```python
from build123d import *

# Parameters (mm, degrees)
F1_DEPTH = 5
F2_R     = 12.5
F3_DEPTH = 3
F3_TAPER = 30
F4_R     = 7.5
F5_DEPTH = 5.0010001
F6_DEPTH = 5.0010001
F7_R     = 3


# Not quite as in the source:
# - a pattern or mirror of a feature is missing from the dataset's text; its kind, count and spacing are read off the source's solid


with BuildPart() as f1:
    # F0 (on Front) → F1 (new body, symmetric)
    with BuildSketch(Plane.XZ):
        with BuildLine():
            ThreePointArc((19.8138622769, -2.7222897845), (19.9534113066, -1.3643229935), (20, 0))
            ThreePointArc((20, 0), (16.5979995869, 11.1582440246), (7.5493590287, 18.5204529711))
            Line((7.5493590287, 18.5204529711), (-7.5493590287, 18.5204529711))
            ThreePointArc((-7.5493590287, 18.5204529711), (-17.3205080757, 10), (-19.8138622769, -2.7222897845))
            Line((-19.8138622769, -2.7222897845), (-12.2645032483, -15.7981631867))
            ThreePointArc((-12.2645032483, -15.7981631867), (0, -20), (12.2645032483, -15.7981631867))
            Line((12.2645032483, -15.7981631867), (19.8138622769, -2.7222897845))
        make_face()
        with BuildLine():
            Line((-7.5493590287, 18.5204529711), (7.5493590287, 18.5204529711))
            ThreePointArc((7.5493590287, 18.5204529711), (0, 20), (-7.5493590287, 18.5204529711))
        make_face()
        with BuildLine():
            ThreePointArc((-7.5493590287, 18.5204529711), (0, 20), (7.5493590287, 18.5204529711))
            Line((7.5493590287, 18.5204529711), (7.5493590287, 42.3402367583))
            Line((7.5493590287, 42.3402367583), (-7.5493590287, 42.3402367583))
            Line((-7.5493590287, 42.3402367583), (-7.5493590287, 18.5204529711))
        make_face()
        with BuildLine():
            Line((40.4424001493, -14.632181678), (19.8138622769, -2.7222897845))
            ThreePointArc((19.8138622769, -2.7222897845), (17.3205080757, -10), (12.2645032483, -15.7981631867))
            Line((12.2645032483, -15.7981631867), (32.8930411206, -27.7080550803))
            Line((32.8930411206, -27.7080550803), (40.4424001493, -14.632181678))
        make_face()
        with BuildLine():
            ThreePointArc((12.2645032483, -15.7981631867), (17.3205080757, -10), (19.8138622769, -2.7222897845))
            Line((19.8138622769, -2.7222897845), (12.2645032483, -15.7981631867))
        make_face()
        with BuildLine():
            Line((-12.2645032483, -15.7981631867), (-19.8138622769, -2.7222897845))
            ThreePointArc((-19.8138622769, -2.7222897845), (-17.3205080757, -10), (-12.2645032483, -15.7981631867))
        make_face()
        with BuildLine():
            ThreePointArc((-12.2645032483, -15.7981631867), (-17.3205080757, -10), (-19.8138622769, -2.7222897845))
            Line((-19.8138622769, -2.7222897845), (-40.4424001493, -14.632181678))
            Line((-40.4424001493, -14.632181678), (-32.8930411206, -27.7080550803))
            Line((-32.8930411206, -27.7080550803), (-12.2645032483, -15.7981631867))
        make_face()
    extrude(amount=F1_DEPTH, both=True)

    # F2 (on face) → F3 (cut)
    with BuildSketch(Plane(origin=(0, 5, 0), x_dir=(-1, 0, 0), z_dir=(0, 1, 0))):
        Circle(F2_R)
    f3 = extrude(amount=-F3_DEPTH, taper=F3_TAPER, mode=Mode.SUBTRACT)

    # F3_copies: F3 across plane
    add(f3.mirror(Plane(origin=(0, 0, 0), x_dir=(0, 0, -1), z_dir=(0, -1, 0))), mode=Mode.SUBTRACT)

    # F4 (on Front) → F5 (cut, through all)
    with BuildSketch(Plane.XZ):
        Circle(F4_R)
    extrude(amount=-F5_DEPTH, mode=Mode.SUBTRACT)

    # F6 (cut, through all): a face of the model
    f6_faces = [f1.faces().sort_by_distance(p)[0] for p in [
        (0, 0, 0),
    ]]
    extrude(f6_faces, amount=-F6_DEPTH, mode=Mode.SUBTRACT)

    # F7
    f7_edges = [f1.edges().sort_by_distance(p)[0] for p in [
        (-7.549359, 0, 42.340237),
        (7.549359, 0, 42.340237),
        (40.4424, 0, -14.632182),
        (32.893041, 0, -27.708055),
        (-32.893041, 0, -27.708055),
        (-40.4424, 0, -14.632182),
    ]]
    fillet(f7_edges, radius=F7_R)


solid = f1.part
```
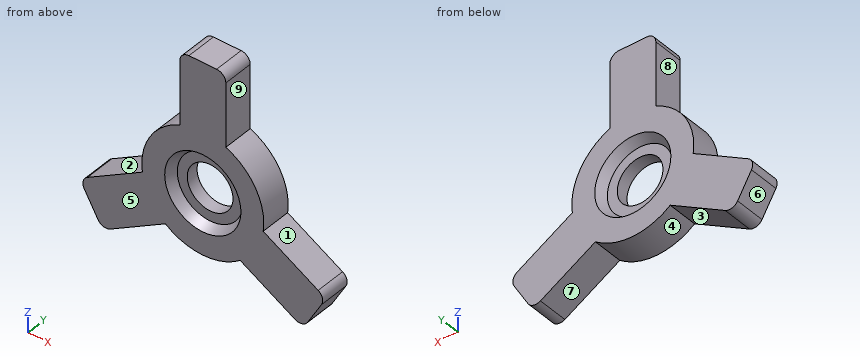
Read the model definition and answer for the solid it produces. Units are mm, in the model's axes. Face numbers are marked on the shaded views. A direction names the side the tool comes from. Round coordinates to 2 decimals unless told otherwise and drop trailing zeros. Write each loop counter-clockwise with the first axis right and the second up, starting at its lowest first coordinate (ties: lowest second). Pieces come first, ordered by that corner, then holes. Notation, with made-up numbers: (78.25, -5) - (132.25, -5) arc R26 ccw to (132.25, 29) - close; hole circle Ø3 at (-15, -33). An arc over 180 degrees is marked (long way). Use CSV: the item, a comma, the result in double quotes.
Q1. Find section B-B, the plane y = -4. Write down the section's boundary in (x, z).
Values:
outline,"(-38.94, -17.23) - (-34.39, -25.11) arc R3 ccw to (-30.29, -26.21) - (-12.26, -15.8) arc R20 ccw to (12.26, -15.8) - (30.29, -26.21) arc R3 ccw to (34.39, -25.11) - (38.94, -17.23) arc R3 ccw to (37.84, -13.13) - (19.81, -2.72) arc R20 ccw to (7.55, 18.52) - (7.55, 39.34) arc R3 ccw to (4.55, 42.34) - (-4.55, 42.34) arc R3 ccw to (-7.55, 39.34) - (-7.55, 18.52) arc R20 ccw to (-19.81, -2.72) - (-37.84, -13.13) arc R3 ccw to start; hole circle Ø23.85 at (0, 0)"
Q2. Find section D-D, the plane y = 3.5. Write down the section's boundary in (x, z).
Values:
outline,"(-38.94, -17.23) - (-34.39, -25.11) arc R3 ccw to (-30.29, -26.21) - (-12.26, -15.8) arc R20 ccw to (12.26, -15.8) - (30.29, -26.21) arc R3 ccw to (34.39, -25.11) - (38.94, -17.23) arc R3 ccw to (37.84, -13.13) - (19.81, -2.72) arc R20 ccw to (7.55, 18.52) - (7.55, 39.34) arc R3 ccw to (4.55, 42.34) - (-4.55, 42.34) arc R3 ccw to (-7.55, 39.34) - (-7.55, 18.52) arc R20 ccw to (-19.81, -2.72) - (-37.84, -13.13) arc R3 ccw to start; hole circle Ø23.27 at (0, 0)"
Q3. Find section A-A, the plane x = 0. Write down the section's boundary in (y, z), then the cut area to 3 significant figures.
Values:
outline,"(-5, -20) - (5, -20) - (5, -12.5) - (2, -10.77) - (2, -7.5) - (-2, -7.5) - (-2, -10.77) - (-5, -12.5) - close; (-5, 12.5) - (-2, 10.77) - (-2, 7.5) - (2, 7.5) - (2, 10.77) - (5, 12.5) - (5, 42.34) - (-5, 42.34) - close"
area,"424 mm²"
Q4. Determine the mould class of the marked faces 1, 2, 3 and 4 for opening direction X: +X half, -X half, draft (parallel to the pull), parting line (faces both ways), or undercut.
Values:
face 1,"+X half"
face 2,"-X half"
face 3,"undercut"
face 4,"undercut"
Q5. Each of these flat-tipped pins is pushed along its axis until it touches: pin 1 Ø3 at (y, z) = (1.5, 27.5) entering from +X; pin 2 Ø5 at (x, z) = (1, -9) entering from -Y; pin 3 Ø2 at (x, y) = (-29, -2.5) entering from +Z. Where does it stop, or does it pass through?
Values:
pin 1,"stops at x = 7.55"
pin 2,"stops at y = -3.36"
pin 3,"stops at z = -7.45"
Q6. Find section C-C, the plane z = 28. Write down the section's boundary in (x, y).
Values:
outline,"(-7.55, -5) - (7.55, -5) - (7.55, 5) - (-7.55, 5) - close"
Q7. A tool of negligible diameter and unlimited length cuts with its end or side. For the marked faces 5, 6, 7, 8 and 9, from which of +Z, -Z, +X, -X, +Y, -Y can it reach the whole face along a straight path? Write none if from no direction.
Values:
face 5,"+Z, -Z, +X, -X, -Y"
face 6,"-Z, -X, +Y, -Y"
face 7,"-Z, +Y, -Y"
face 8,"+Z, -X, +Y, -Y"
face 9,"+Z, +X, +Y, -Y"
Q8. Straight lines are drawn through the part: line 1 along Z through (x, y) = (0, 0); line 2 along X through (y, z) = (-3, 31); line 3 along Z through (x, y) = (5, -0.25). For each, find the intervals that lie inside material, in ascending order.
Values:
line 1,"z = -20 to -7.5, 7.5 to 42.34"
line 2,"x = -7.55 to 7.55"
line 3,"z = -19.36 to -5.59, 5.59 to 42.31"
